Can you work these out from the drawing? Everything is in mm from the part's minimum corner. A direction names the side the tool comes from. Coordinates: 2 decimals unless noted, no trailing zeros. Loops run counter-clockwise (first coordinate to the right, second up) from the corner with the lowest first, then second, coordinate; pieces in that order, holes last. Notation, with made-up numbers: (25.25, 9) - (30.25, 9) arc R20 ccw to (30.25, 33) - close; hole circle Ø9 at (-27.5, -30.75). An arc over 180 degrees is marked (long way). One line per question, with ' | ' between items. Start each with the question number.
1. I want a section at B-B, the plane x = 5.25. Write out the boundary of the cut face in (y, z), then the cut area to 3 significant figures.
2. Which directions (+Z, -Z, +X, -X, +Y, -Y) give clear straight access to the entire face, cutting with the end or side of a thin tool? Please do the marked faces 1, 2 and 3.
3. Please list where these lines run through material, in increasing order: L1, parallel to Y at x = 4.25, z = 7.5; L2, parallel to Y at x = 1.75, z = 2.5; L3, parallel to Z at x = 0.5, y = 27. Write a range as [from, to].
4. I want a section at A-A, the plane y = 26. Write out the boundary of the cut face in (x, z), then the cut area to 3 significant figures.
5. I'm going to push a flat-ended pin straight in: P1, Ø5, axis at x = 5.5, z = 7.5, coming from the +Y side. Where does the tip first touch, or does it pass through?
6. I want a section at C-C, the plane z = 4.5. Write out the boundary of the cut face in (x, y).
7. I want a section at D-D, the plane x = 1. Write out the boundary of the cut face in (y, z), then the cut area to 3 significant figures.
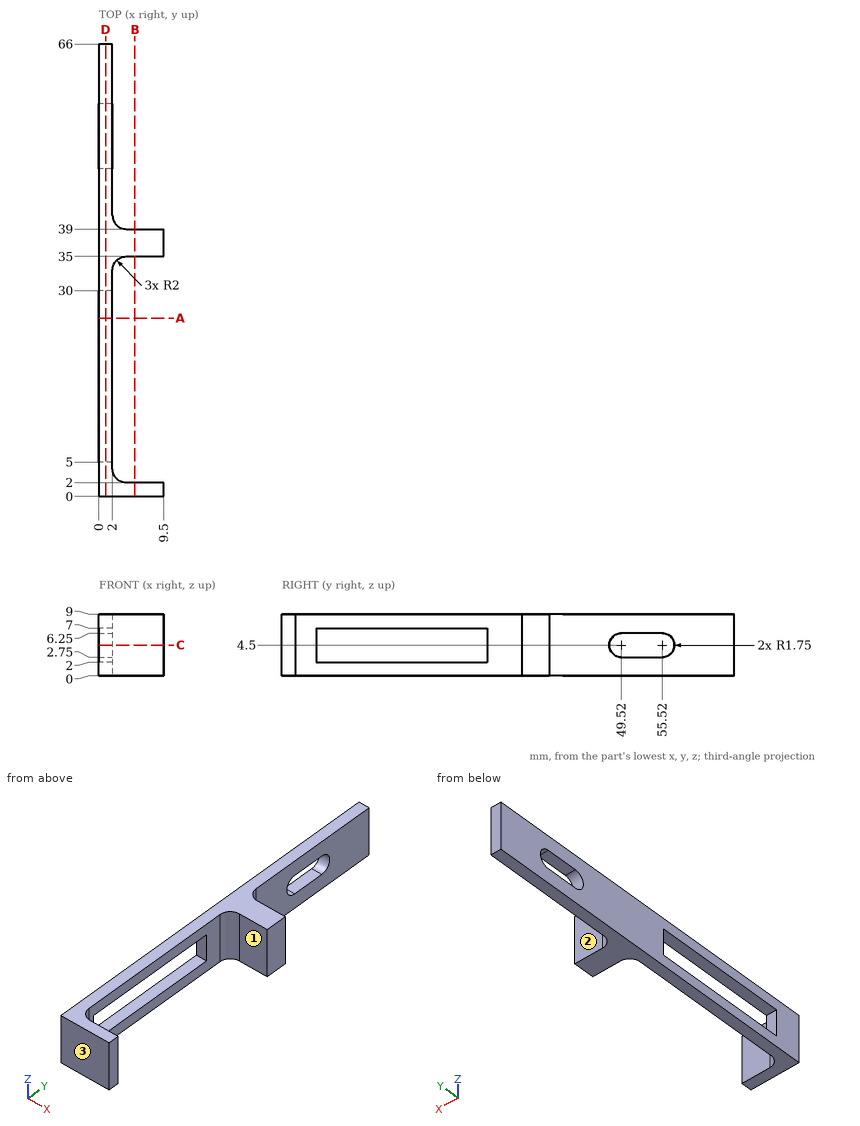
Results are:
1) outline: (0, 0) - (2, 0) - (2, 9) - (0, 9) - close; (35, 0) - (39, 0) - (39, 9) - (35, 9) - close | area: 54.0 mm2
2) face 1: +Z, -Z, +X | face 2: +Z, -Z, +X, +Y | face 3: +Z, -Z, +X, -X, -Y
3) L1: y = [0, 2], [35, 39] | L2: y = [0, 5], [30, 66] | L3: z = [0, 2], [7, 9]
4) outline: (0, 0) - (2, 0) - (2, 2) - (0, 2) - close; (0, 7) - (2, 7) - (2, 9) - (0, 9) - close | area: 8.00 mm2
5) P1: stops at y = 39.27
6) outline: (0, 0) - (9.5, 0) - (9.5, 2) - (4, 2) arc R2 cw to (2, 4) - (2, 5) - (0, 5) - close; (0, 30) - (2, 30) - (2, 33) arc R2 cw to (4, 35) - (9.5, 35) - (9.5, 39) - (4, 39) arc R2 cw to (2, 41) - (2, 47.77) - (0, 47.77) - close; (0, 57.27) - (2, 57.27) - (2, 66) - (0, 66) - close
7) outline: (0, 0) - (66, 0) - (66, 9) - (0, 9) - close; hole (5, 2) - (30, 2) - (30, 7) - (5, 7) - close; hole (49.52, 2.75) - (55.52, 2.75) arc R1.75 ccw to (55.52, 6.25) - (49.52, 6.25) arc R1.75 ccw to start | area: 438 mm2
